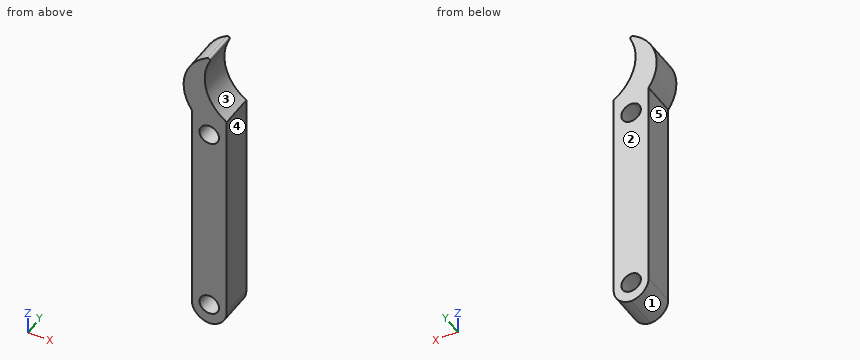
```python
from build123d import *

# Parameters (mm, degrees)
SKETCH1_R           = 2.667
BOSS_EXTRUDE1_DEPTH = 9.525
FILLET1_R           = 5.08
FILLET2_R           = 0.508


with BuildPart() as part:
    # Sketch1 → Boss-Extrude1 (new body)
    with BuildSketch(Plane(origin=(0, 0, 0), x_dir=(1, 0, 0), z_dir=(0, 1, 0))):
        with BuildLine():
            Line((-4.7625, 31.75), (4.7625, 31.75))
            Line((4.7625, 31.75), (4.7625, -31.75))
            ThreePointArc((4.7625, -31.75), (-0.950597142, -40.049292778), (0.9525, -49.943531548))
            ThreePointArc((0.9525, -49.943531548), (-6.432834073, -42.269060926), (-4.7625, -31.75))
            Line((-4.7625, -31.75), (-4.7625, 31.75))
        make_face()
        with Locations(Location((0, -26.035, 0), (0, 0, 90))):
            Circle(SKETCH1_R, mode=Mode.SUBTRACT)
        with Locations(Location((0, 26.035, 0), (0, 0, 90))):
            Circle(SKETCH1_R, mode=Mode.SUBTRACT)
    extrude(amount=BOSS_EXTRUDE1_DEPTH)

    # Fillet1
    # the kernel refuses this fillet: 5.08 mm, written as the material it takes off along each edge
    with BuildSketch(Plane(origin=(-4.7625, -12.7, -31.75), x_dir=(0, 0, 1), z_dir=(0, 1, 0)), Plane(origin=(4.7625, -12.7, -31.75), x_dir=(-1, 0, 0), z_dir=(0, 1, 0))) as fillet1_piece_1:
        with BuildLine():
            CenterArc((FILLET1_R, FILLET1_R), FILLET1_R, 180, 90)
            Line((0, FILLET1_R), (0, 0))
            Line((0, 0), (FILLET1_R, 0))
        make_face()
    extrude(amount=34.925, mode=Mode.SUBTRACT)

    # Fillet2
    fillet2_edges = [part.edges().sort_by_distance(p)[0] for p in [
        (0.9525, 4.7625, 49.943531548),
    ]]
    fillet(fillet2_edges, radius=FILLET2_R)


solid = part.part
```
Work out the finished part from the listing and answer in its coordinate system (mm). Face numbers are marked on the shaded views. A direction names the side the tool comes from. Give positions to 0.01 mm unless a question says otherwise; leave off trailing zeros. Write each loop counter-clockwise with the first axis right and the second up, starting at its lowest first coordinate (ties: lowest second). Pieces come first, ordered by that corner, then holes. Notation, with made-up numbers: (42, -12) - (97, -12) arc R13 ccw to (97, 13) - close; hole circle Ø11 at (-5.5, 69). An arc over 180 degrees is marked (long way). Use one line per item in the form item = value.
1. A cutting plane is placed at A-A (x = -2). Write down the section's boundary in (y, z) (3 decimals).
Filled in:
outline = (0, -31.191) - (9.525, -31.191) - (9.525, -27.799) - (0, -27.799) - close; (0, -24.271) - (9.525, -24.271) - (9.525, 24.271) - (0, 24.271) - close; (0, 27.799) - (9.525, 27.799) - (9.525, 48.396) - (0, 48.396) - close
2. Determine the mould class of the marked faces 1, 2 and 3 for opening direction Z: released by +Z, released by -Z, zero draft, split by the parting line, or undercut.
Filled in:
face_1 = released by -Z
face_2 = zero draft
face_3 = undercut
3. A cutting plane is placed at D-D (y = 7). State how many separate pieces and enclosed holes the cut face has, and give its area (3 significant figures).
Filled in:
separate_pieces = 1
enclosed_holes = 2
area = 649 mm^2
4. A cutting plane is placed at C-C (z = -20.5). Write down the section's boundary in (x, y) (1 decimal), and give its area (3 significant figures).
Filled in:
outline = (-4.8, 0) - (4.8, 0) - (4.8, 9.5) - (-4.8, 9.5) - close
area = 90.7 mm^2
5. Consider L1, parallel to X at y = 7, z = 29; L2, parallel to Z at x = 0.75, y = 6; L3, parallel to Z at x = -0.25, y = 7.25. Determine where each line is inside the solid, lowest interval first.
Filled in:
L1 = -4.76 to 4.76
L2 = -31.64 to -28.59, -23.48 to 23.48, 28.59 to 35.82
L3 = -31.72 to -28.69, -23.38 to 23.38, 28.69 to 37.77, 47.68 to 49.37
6. A cutting plane is placed at B-B (z = 24.5). Write down the section's boundary in (x, y) (1 decimal).
Filled in:
outline = (-4.8, 0) - (-2.2, 0) - (-2.2, 9.5) - (-4.8, 9.5) - close; (2.2, 0) - (4.8, 0) - (4.8, 9.5) - (2.2, 9.5) - close
7. For the marked faces 4 and 5, determine the directions among +Z, -Z, +X, -X, +Y, -Y from which every point of the face is accessible in a straight line to the end or side of a thin tool.
Filled in:
face_4 = +Z, -Z, +X, +Y, -Y
face_5 = -Z, -X, +Y, -Y
8. Each of these flat-tipped pins is pushed along its axis until it touches: pin 1 Ø4 at (x, y) = (-4, 4.5) entering from +Z; pin 2 Ø3 at (y, z) = (6.5, -2) entering from -X; pin 3 Ø1 at (x, y) = (3, 6.5) entering from -Z. Where does it stop, or does it pass through?
Filled in:
pin_1 = 48.4
pin_2 = -4.76
pin_3 = -30.9
